```python
from build123d import *

# Parameters (mm, degrees)
SKETCH1_R           = 2.95
BOSS_EXTRUDE1_DEPTH = 22.686
SKETCH3_W           = 6.9
SKETCH3_H           = 5.9
BOSS_EXTRUDE2_DEPTH = 8
FILLET1_R           = 2.54
FILLET2_R           = 0.75
BOSS_EXTRUDE3_START = -8
SKETCH4_W           = 2.032
SKETCH4_H           = 2.032
BOSS_EXTRUDE3_DEPTH = 2


with BuildPart() as part:
    # Sketch1 → Boss-Extrude1 (new body)
    with BuildSketch(Plane(origin=(0, 0, 0), x_dir=(1, 0, 0), z_dir=(0, 1, 0))):
        Circle(SKETCH1_R)
    extrude(amount=BOSS_EXTRUDE1_DEPTH)

    # Sketch3 → Boss-Extrude2 (add)
    with BuildSketch(Plane(origin=(0, 22.686, 0), x_dir=(1, 0, 0), z_dir=(0, 1, 0))):
        Rectangle(SKETCH3_W, SKETCH3_H)
    extrude(amount=BOSS_EXTRUDE2_DEPTH)

    # Fillet1
    fillet1_edges = [part.edges().sort_by_distance(p)[0] for p in [
        (3.45, 26.686, 2.95),
        (3.45, 26.686, -2.95),
        (-3.45, 26.686, -2.95),
        (-3.45, 26.686, 2.95),
    ]]
    fillet(fillet1_edges, radius=FILLET1_R)

    # Fillet2
    fillet2_edges = [part.edges().sort_by_distance(p)[0] for p in [
        (-3.45, 30.686, 0),
        (0, 30.686, -2.95),
        (3.45, 30.686, 0),
        (0, 30.686, 2.95),
        (-2.706051224, 30.686, 2.206051224),
        (2.706051224, 30.686, 2.206051224),
        (2.706051224, 30.686, -2.206051224),
        (-2.706051224, 30.686, -2.206051224),
    ]]
    fillet(fillet2_edges, radius=FILLET2_R)

    # Sketch4 → Boss-Extrude3 (add)
    with BuildSketch(Plane(origin=(0, 30.686, 0), x_dir=(1, 0, 0), z_dir=(0, 1, 0)).offset(BOSS_EXTRUDE3_START)):
        with Locations((0, 3.966)):
            Rectangle(SKETCH4_W, SKETCH4_H)
        with Locations((0, -3.966)):
            Rectangle(SKETCH4_W, SKETCH4_H)
    extrude(amount=BOSS_EXTRUDE3_DEPTH)


solid = part.part
```
Source: CAD feature listing. Evaluate the final solid. Frame: model axes, mm. A direction names the side the tool comes from. Coordinates: 2 decimals unless noted, no trailing zeros. Write each loop counter-clockwise with the first axis right and the second up, starting at its lowest first coordinate (ties: lowest second). Pieces come first, ordered by that corner, then holes. Notation, with made-up numbers: M 13.5,46 L 31.5,46 A16 ccw 31.5,58 Z; hole C 34.5,45.25 d10. An arc over 180 degrees is marked long. Answer as a JSON object with one key per item and string values.
1. Cut plane A-A on y = 23. Output: boundary loops of the cut face in (x, z), plus the area to 3 significant figures.
Evaluation:
{"outline": "M -3.45,-0.41 A2.54 ccw -0.91,-2.95 L -1.02,-2.95 L -1.02,-4.98 L 1.02,-4.98 L 1.02,-2.95 L 0.91,-2.95 A2.54 ccw 3.45,-0.41 L 3.45,0.41 A2.54 ccw 0.91,2.95 L 1.02,2.95 L 1.02,4.98 L -1.02,4.98 L -1.02,2.95 L -0.91,2.95 A2.54 ccw -3.45,0.41 Z", "area": "43.4 mm^2"}
2. Contact query for flat-ended pins moving along their axis: P1, Ø0.6, axis at y = 23.5, z = 3.5, coming from the +X side; P2, Ø1.6, axis at x = -0.5, z = 4.5, coming from the +Y side; P3, Ø1, axis at y = 27, z = -1, coming from the -X side; P4, Ø0.6, axis at y = 24, z = 4, coming from the -X side. Output: stop coordinate, or through.
Evaluation:
{"P1": "x = 1.02", "P2": "y = 24.69", "P3": "x = -3.45", "P4": "x = -1.02"}
3. Cut plane C-C on z = 0. Output: boundary loops of the cut face in (x, y), plus the area to 3 significant figures.
Evaluation:
{"outline": "M -3.45,22.69 L -2.95,22.69 L -2.95,0 L 2.95,0 L 2.95,22.69 L 3.45,22.69 L 3.45,29.94 A0.75 ccw 2.7,30.69 L -2.7,30.69 A0.75 ccw -3.45,29.94 Z", "area": "189 mm^2"}
4. Ray query, L1, parallel to Y at x = 0, z = 2.25; L2, parallel to Z at x = -0.75, y = 28.5; L3, parallel to X at y = 23, z = -0.5. Return the intervals inside material, ascending.
Evaluation:
{"L1": "0 to 30.68", "L2": "-2.95 to 2.95", "L3": "-3.45 to 3.45"}
5. Cut plane D-D on y = 12. Output: boundary loops of the cut face in (x, z).
Evaluation:
{"outline": "C 0,0 d5.9"}
6. Access query for faces 1 (the flat face through (1.016, 24, -4)), 2 (the flat face through (0, 27, 2.95)), 3 (the cylindrical face through (-2.947, 11.184, -0.13)), 4 (the flat face through (1.016, 24, 4)). Directions: +Z, -Z, +X, -X, +Y, -Y. A direction counts if a zero-diameter tool reaches every point of the face in a straight line with its end or side. Return the directions, or none.
Evaluation:
{"face 1": "-Z, +X, +Y, -Y", "face 2": "+Z, +X, -X, +Y", "face 3": "-Y", "face 4": "+Z, +X, +Y, -Y"}
7. Cut plane B-B on x = 0. Output: boundary loops of the cut face in (y, z).
Evaluation:
{"outline": "M 0,-2.95 L 22.69,-2.95 L 22.69,-4.98 L 24.69,-4.98 L 24.69,-2.95 L 29.94,-2.95 A0.75 ccw 30.69,-2.2 L 30.69,2.2 A0.75 ccw 29.94,2.95 L 24.69,2.95 L 24.69,4.98 L 22.69,4.98 L 22.69,2.95 L 0,2.95 Z"}
